from build123d import *

# Parameters (mm, degrees)
SKETCH_1_R          = 11
SKETCH_1_R_2        = 4
EXTRUDE_1_DEPTH     = 3.5
CUT_EXTRUDE_START   = 3.5
SKETCH_2_R          = 9.5
SKETCH_2_R_2        = 6
CUT_EXTRUDE_1_DEPTH = 0.4


with BuildPart() as part:
    # 草圖1 → 填料-伸長1 (new body, symmetric)
    with BuildSketch(Plane(origin=(0, 0, 0), x_dir=(1, 0, 0), z_dir=(0, 1, 0))):
        Circle(SKETCH_1_R)
        Circle(SKETCH_1_R_2, mode=Mode.SUBTRACT)
    extrude(amount=EXTRUDE_1_DEPTH, both=True)

    # 草圖2 → 除料-伸長1 (cut)
    with BuildSketch(Plane(origin=(0, 0, 0), x_dir=(1, 0, 0), z_dir=(0, 1, 0)).offset(CUT_EXTRUDE_START)):
        Circle(SKETCH_2_R)
        Circle(SKETCH_2_R_2, mode=Mode.SUBTRACT)
    cut_extrude_1 = extrude(amount=-CUT_EXTRUDE_1_DEPTH, mode=Mode.SUBTRACT)

    # 鏡射4: 除料-伸長1 across plane
    add(cut_extrude_1.mirror(Plane.ZX), mode=Mode.SUBTRACT)


solid = part.part
Work out the finished part from the listing and answer in its coordinate system (mm). A direction names the side the tool comes from. Round coordinates to 2 decimals unless told otherwise and drop trailing zeros. Order: outer loops, then holes, each group sorted by start corner. A loop starts at its lowest first (then second) coordinate and runs counter-clockwise, first axis right, second up. Notation, with made-up numbers: M 22.25,42 L 80.25,42 A19 ccw 80.25,58 Z; hole C -29.75,53.5 d5. An arc over 180 degrees is marked long. One line per item, written item: value.
Q1. Find section B-B on z = 0. Write down the section's boundary in (x, y), then the cut area to 3 significant figures.
Derived:
outline: M -11,-3.5 L -9.5,-3.5 L -9.5,-3.1 L -6,-3.1 L -6,-3.5 L -4,-3.5 L -4,3.5 L -6,3.5 L -6,3.1 L -9.5,3.1 L -9.5,3.5 L -11,3.5 Z; M 4,-3.5 L 6,-3.5 L 6,-3.1 L 9.5,-3.1 L 9.5,-3.5 L 11,-3.5 L 11,3.5 L 9.5,3.5 L 9.5,3.1 L 6,3.1 L 6,3.5 L 4,3.5 Z
area: 92.4 mm²
Q2. Flat-ended cylindrical pins translate along their axes: pin 1 (9.5 mm diameter, centred on x = 1, z = -2, fed in from +Y); pin 2 (2 mm diameter, centred on x = 6.5, y = 1.5, fed in from -Z); pin 3 (4 mm diameter, centred on y = -2.5, z = -7.5, fed in from +X); pin 4 (5 mm diameter, centred on x = 0, z = 0, fed in from -Y). Find the tip coordinate at first contact, or state that the pin passes through.
Derived:
pin 1: y = 3.5
pin 2: z = -9.53
pin 3: x = 9.53
pin 4: through
Q3. Determine the mould class of faces 1 (the face through (-2.38, 0.05, 10.74)), 2 (the face through (-10, 3.5, 0)), 3 (the face through (4.38, 3.3, 8.43)) for opening direction X: released by +X, released by -X, zero draft, split by the parting line, or undercut.
Derived:
face 1: split by the parting line
face 2: zero draft
face 3: undercut
Q4. Straight lines are drawn through the part: line 1 (X direction, y = 3.4, z = 0); line 2 (Z direction, x = 0, y = 0.5). For each, find the intervals that lie inside material, in ascending order.
Derived:
line 1: -11 to -9.5, -6 to -4, 4 to 6, 9.5 to 11
line 2: -11 to -4, 4 to 11
Q5. Find section C-C on x = -6.75. Write down the section's boundary in (y, z), then the cut area to 3 significant figures.
Derived:
outline: M -3.5,-8.69 L 3.5,-8.69 L 3.5,-6.68 L 3.1,-6.68 L 3.1,6.68 L 3.5,6.68 L 3.5,8.69 L -3.5,8.69 L -3.5,6.68 L -3.1,6.68 L -3.1,-6.68 L -3.5,-6.68 Z
area: 111 mm²
Q6. Find section D-D on y = -0.75. Write down the section's boundary in (x, z), then the cut area to 3 significant figures.
Derived:
outline: C 0,0 d22; hole C 0,0 d8
area: 330 mm²
Q7. For faces 4 (the face through (-0.1, 3.1, 6.2)), 5 (the face through (-10, -3.5, 0)), 6 (the face through (4.38, -3.3, 8.43)), determine the directions among +Z, -Z, +X, -X, +Y, -Y from which every point of the face is accessible in a straight line to the end or side of a thin tool.
Derived:
face 4: +Y
face 5: +Z, -Z, +X, -X, -Y
face 6: -Y
Q8. Find section A-A on x = 0. Write down the section's boundary in (y, z).
Derived:
outline: M -3.5,-11 L 3.5,-11 L 3.5,-9.5 L 3.1,-9.5 L 3.1,-6 L 3.5,-6 L 3.5,-4 L -3.5,-4 L -3.5,-6 L -3.1,-6 L -3.1,-9.5 L -3.5,-9.5 Z; M -3.5,4 L 3.5,4 L 3.5,6 L 3.1,6 L 3.1,9.5 L 3.5,9.5 L 3.5,11 L -3.5,11 L -3.5,9.5 L -3.1,9.5 L -3.1,6 L -3.5,6 Z
